from build123d import *

# Parameters (mm, degrees)
ESBO_O1_W                  = 300
ESBO_O1_H                  = 25
RESSALTO_EXTRUS_O1_DEPTH   = 50
FILETE1_R                  = 4
FILETE2_R                  = 15
CORTE_EXTRUS_O2_DEPTH      = 159.607219382
CORTE_EXTRUS_O2_DEPTH_BACK = 159.607219382
ESBO_O8_R                  = 7.5


with BuildPart() as part:
    # Esboço1 → Ressalto-extrusão1 (new body)
    with BuildSketch(Plane(origin=(0, 0, 0), x_dir=(0, 0, -1), z_dir=(1, 0, 0))):
        Rectangle(ESBO_O1_W, ESBO_O1_H)
    extrude(amount=RESSALTO_EXTRUS_O1_DEPTH)

    # Filete1
    filete1_edges = [part.edges().sort_by_distance(p)[0] for p in [
        (50, 12.5, 0),
        (0, 12.5, 0),
        (25, 12.5, 150),
        (25, 12.5, -150),
    ]]
    fillet(filete1_edges, radius=FILETE1_R)

    # Filete2
    # the kernel refuses this fillet: 15 mm, written as the material it takes off along each edge
    with BuildSketch(Plane(origin=(35, 12.5, 135), x_dir=(0, 0, 1), z_dir=(-1, 0, 0))) as filete2_piece_1:
        with BuildLine():
            CenterArc((11, -4), 4, 0, 90)
            Line((15, -4), (15, 0))
            Line((15, 0), (11, 0))
        make_face()
    revolve(axis=Axis((35, 12.5, 135), (0, 1, 0)), revolution_arc=90, mode=Mode.SUBTRACT)
    with BuildSketch(Plane(origin=(15, 12.5, 135), x_dir=(-1, 0, 0), z_dir=(0, 0, -1))) as filete2_piece_2:
        with BuildLine():
            CenterArc((11, -4), 4, 0, 90)
            Line((15, -4), (15, 0))
            Line((15, 0), (11, 0))
        make_face()
    revolve(axis=Axis((15, 12.5, 135), (0, 1, 0)), revolution_arc=90, mode=Mode.SUBTRACT)
    with BuildSketch(Plane(origin=(35, 12.5, -135), x_dir=(1, 0, 0), z_dir=(0, 0, 1))) as filete2_piece_3:
        with BuildLine():
            CenterArc((11, -4), 4, 0, 90)
            Line((15, -4), (15, 0))
            Line((15, 0), (11, 0))
        make_face()
    revolve(axis=Axis((35, 12.5, -135), (0, 1, 0)), revolution_arc=90, mode=Mode.SUBTRACT)
    with BuildSketch(Plane(origin=(15, 12.5, -135), x_dir=(0, 0, -1), z_dir=(1, 0, 0))) as filete2_piece_4:
        with BuildLine():
            CenterArc((11, -4), 4, 0, 90)
            Line((15, -4), (15, 0))
            Line((15, 0), (11, 0))
        make_face()
    revolve(axis=Axis((15, 12.5, -135), (0, 1, 0)), revolution_arc=90, mode=Mode.SUBTRACT)
    with BuildSketch(Plane(origin=(50, 12.5, 150), x_dir=(0, 0, -1), z_dir=(0, -1, 0)), Plane(origin=(0, -50, -150), x_dir=(1, 0, 0), z_dir=(0, 1, 0))) as filete2_piece_5:
        with BuildLine():
            CenterArc((FILETE2_R, -FILETE2_R), FILETE2_R, 90, 90)
            Line((0, -FILETE2_R), (0, 0))
            Line((0, 0), (FILETE2_R, 0))
        make_face()
    extrude(amount=62.5, mode=Mode.SUBTRACT)
    with BuildSketch(Plane(origin=(0, 12.5, 150), x_dir=(0, 0, -1), z_dir=(0, -1, 0)), Plane(origin=(50, -50, -150), x_dir=(-1, 0, 0), z_dir=(0, 1, 0))) as filete2_piece_6:
        with BuildLine():
            CenterArc((FILETE2_R, FILETE2_R), FILETE2_R, 180, 90)
            Line((0, FILETE2_R), (0, 0))
            Line((0, 0), (FILETE2_R, 0))
        make_face()
    extrude(amount=62.5, mode=Mode.SUBTRACT)

    # Esboço8 → Corte-extrusão2 (cut, two sides: drawn at the far end of the back side and taken through both)
    with BuildSketch(Plane.XY.offset(-CORTE_EXTRUS_O2_DEPTH_BACK)):
        with Locations((24.323943137, -12.5)):
            Circle(ESBO_O8_R)
    extrude(amount=CORTE_EXTRUS_O2_DEPTH + CORTE_EXTRUS_O2_DEPTH_BACK, mode=Mode.SUBTRACT)


solid = part.part
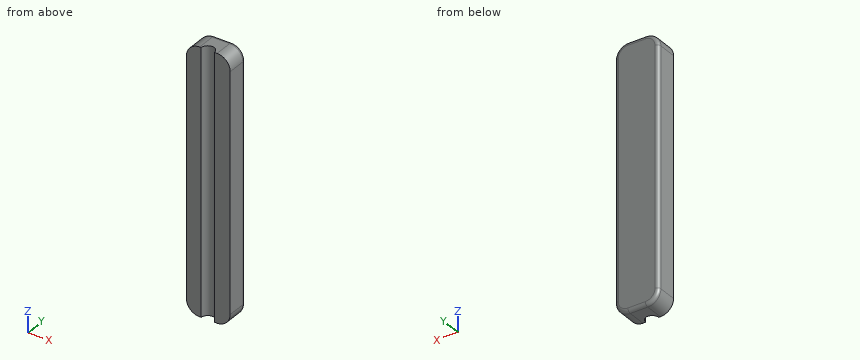
Model file for the job. Use its own axes, mm. Give positions to 0.01 mm unless a question says otherwise; leave off trailing zeros. Order: outer loops, then holes, each group sorted by start corner. A loop starts at its lowest first (then second) coordinate and runs counter-clockwise, first axis right, second up. Notation, with made-up numbers: (-14, 18) - (36, 18) arc R20 ccw to (36, 44) - close; hole circle Ø3 at (64.25, 54.25). An arc over 180 degrees is marked (long way). Return JSON: item names as keys, results as strings.
1) Flat gauge pins, fed straight in: P1, Ø6, axis at x = 10.5, y = 5, coming from the -Z side; P2, Ø1.5, axis at x = 19, y = -9.5, coming from the +Z side; P3, Ø2, axis at x = 8, y = -1, coming from the +Z side; P4, Ø4, axis at x = 38, y = 1.5, coming from the +Z side. Where does each tip first touch, or does it go through?
Geometry says:
{"P1": "z = -149.92", "P2": "through", "P3": "z = 148.75", "P4": "z = 149.97"}
2) Cut at A-A, the plane y = -10. Give the cut face in (x, z), plus the area to 3 significant figures.
Geometry says:
{"outline": "(0, -135) arc R15 ccw to (15, -150) - (17.25, -150) - (17.25, 150) - (15, 150) arc R15 ccw to (0, 135) - close; (31.4, -150) - (35, -150) arc R15 ccw to (50, -135) - (50, 135) arc R15 ccw to (35, 150) - (31.4, 150) - close", "area": "10,600 mm²"}
3) Probe line 1 (Y direction, x = 25, z = -108); line 2 (X direction, y = -5.75, z = 38.5); line 3 (X direction, y = -6.5, z = 73.5). List the from-to ranges inside material, lowest first. Write a range as from..to.
Geometry says:
{"line 1": "-5.03..12.5", "line 2": "0..21.05, 27.59..50", "line 3": "0..19.82, 28.82..50"}
4) Cut at C-C, the plane x = 25. Give the cut face in (y, z).
Geometry says:
{"outline": "(-5.03, -150) - (8.5, -150) arc R4 ccw to (12.5, -146) - (12.5, 146) arc R4 ccw to (8.5, 150) - (-5.03, 150) - close"}
5) Cut at B-B, the plane z = 34. Give the cut face in (x, y), plus the area to 3 significant figures.
Geometry says:
{"outline": "(0, -12.5) - (16.82, -12.5) arc R7.5 cw to (31.82, -12.5) - (50, -12.5) - (50, 8.5) arc R4 ccw to (46, 12.5) - (4, 12.5) arc R4 ccw to (0, 8.5) - close", "area": "1,150 mm²"}
